from build123d import *

# Parameters (mm, degrees)
F1_DEPTH = 2
F2_DEPTH = 8
F3_DEPTH = 7.25


with BuildPart() as f1:
    # F0 (on Top) → F1 (new body)
    with BuildSketch(Plane.XY):
        with BuildLine():
            Line((4.85, 7.2), (-4.85, 7.2))
            ThreePointArc((-4.85, 7.2), (-6.5117009358, 6.5117009358), (-7.2, 4.85))
            Line((-7.2, 4.85), (-7.2, -4.85))
            ThreePointArc((-7.2, -4.85), (-6.5117009358, -6.5117009358), (-4.85, -7.2))
            Line((-4.85, -7.2), (4.85, -7.2))
            ThreePointArc((4.85, -7.2), (6.5117009358, -6.5117009358), (7.2, -4.85))
            Line((7.2, -4.85), (7.2, 4.85))
            ThreePointArc((7.2, 4.85), (6.5117009358, 6.5117009358), (4.85, 7.2))
        make_face()
        with BuildLine():
            ThreePointArc((6.45, -4.85), (5.9813708499, -5.9813708499), (4.85, -6.45))
            Line((4.85, -6.45), (-4.85, -6.45))
            ThreePointArc((-4.85, -6.45), (-5.9813708499, -5.9813708499), (-6.45, -4.85))
            Line((-6.45, -4.85), (-6.45, 4.85))
            ThreePointArc((-6.45, 4.85), (-5.9813708499, 5.9813708499), (-4.85, 6.45))
            Line((-4.85, 6.45), (4.85, 6.45))
            ThreePointArc((4.85, 6.45), (5.9813708499, 5.9813708499), (6.45, 4.85))
            Line((6.45, 4.85), (6.45, -4.85))
        make_face(mode=Mode.SUBTRACT)
    extrude(amount=F1_DEPTH)

    # F0 (on Top) → F2 (join)
    with BuildSketch(Plane.XY):
        with BuildLine():
            Line((-4.85, -6.45), (4.85, -6.45))
            ThreePointArc((4.85, -6.45), (5.9813708499, -5.9813708499), (6.45, -4.85))
            Line((6.45, -4.85), (6.45, 4.85))
            ThreePointArc((6.45, 4.85), (5.9813708499, 5.9813708499), (4.85, 6.45))
            Line((4.85, 6.45), (-4.85, 6.45))
            ThreePointArc((-4.85, 6.45), (-5.9813708499, 5.9813708499), (-6.45, 4.85))
            Line((-6.45, 4.85), (-6.45, -4.85))
            ThreePointArc((-6.45, -4.85), (-5.9813708499, -5.9813708499), (-4.85, -6.45))
        make_face()
        Polygon((1.355533, 3.320697), (-0.67179, 0.676571), (-0.439293, 0.773395), (-0.210383, 0.843921), (0.016137, 0.886954), (0.241462, 0.901298), (0.470596, 0.891361), (0.689421, 0.861552), (0.897936, 0.81187), (1.096141, 0.742316), (1.284036, 0.652888), (1.461621, 0.543588), (1.628896, 0.414415), (1.785861, 0.265369), (1.928183, 0.100858), (2.051528, -0.07471), (2.155898, -0.261335), (2.241291, -0.459016), (2.307708, -0.667755), (2.355149, -0.887551), (2.383613, -1.118404), (2.393101, -1.360314), (2.382455, -1.62389), (2.350517, -1.874317), (2.297286, -2.111595), (2.222763, -2.335724), (2.126948, -2.546704), (2.00984, -2.744536), (1.871441, -2.929218), (1.711749, -3.100751), (1.534649, -3.2554), (1.344027, -3.38943), (1.139883, -3.502839), (0.922217, -3.595628), (0.691027, -3.667798), (0.446316, -3.719348), (0.188082, -3.750277), (-0.083675, -3.760587), (-0.337875, -3.750502), (-0.579299, -3.720244), (-0.807948, -3.669815), (-1.023822, -3.599214), (-1.22692, -3.508442), (-1.417243, -3.397498), (-1.594791, -3.266383), (-1.759563, -3.115096), (-1.908048, -2.947372), (-2.036736, -2.766948), (-2.145625, -2.573824), (-2.234717, -2.367999), (-2.30401, -2.149473), (-2.353505, -1.918246), (-2.383202, -1.674319), (-2.393101, -1.417691), (-2.387124, -1.273221), (-2.369194, -1.12072), (-2.33931, -0.960188), (-2.297473, -0.791624), (-2.243682, -0.615029), (-2.177937, -0.430403), (-2.100239, -0.237745), (-2.010587, -0.037056), (-1.795423, 0.388416), (-1.532445, 0.846013), (-1.221653, 1.335735), (-0.863046, 1.857582), (-0.73873, 2.024932), (0.485314, 3.760587), align=None, mode=Mode.SUBTRACT)
    extrude(amount=F2_DEPTH)



with BuildPart() as f2:
    # F0 (on Top) → F2, piece 2 (new body)
    with BuildSketch(Plane.XY):
        Polygon((-1.302227, -1.275519), (-1.307719, -1.427254), (-1.302265, -1.580035), (-1.285903, -1.725196), (-1.258634, -1.862737), (-1.220458, -1.992657), (-1.171373, -2.114957), (-1.111381, -2.229636), (-1.040482, -2.336695), (-0.958675, -2.436134), (-0.868201, -2.525786), (-0.771303, -2.603484), (-0.667979, -2.669228), (-0.558231, -2.723019), (-0.442057, -2.764857), (-0.319459, -2.79474), (-0.190435, -2.812671), (-0.054986, -2.818648), (0.097421, -2.81282), (0.241462, -2.795338), (0.377135, -2.766201), (0.50444, -2.72541), (0.623378, -2.672964), (0.733948, -2.608863), (0.836151, -2.533107), (0.929986, -2.445697), (1.014035, -2.348201), (1.086877, -2.242188), (1.148512, -2.127658), (1.198941, -2.004611), (1.238164, -1.873047), (1.26618, -1.732966), (1.28299, -1.584369), (1.288593, -1.427254), (1.283064, -1.267936), (1.266479, -1.117508), (1.238836, -0.97597), (1.200137, -0.843323), (1.15038, -0.719566), (1.089566, -0.6047), (1.017696, -0.498725), (0.934768, -0.401639), (0.842053, -0.314789), (0.740821, -0.239519), (0.631073, -0.175829), (0.512807, -0.123719), (0.386025, -0.083189), (0.250726, -0.054239), (0.10691, -0.036869), (-0.045423, -0.031079), (-0.18203, -0.037131), (-0.312137, -0.055285), (-0.435744, -0.085543), (-0.552852, -0.127903), (-0.663459, -0.182366), (-0.767567, -0.248933), (-0.865176, -0.327602), (-0.956284, -0.418374), (-1.038652, -0.518859), (-1.110037, -0.626665), (-1.17044, -0.741793), (-1.21986, -0.864242), (-1.258298, -0.994013), (-1.285754, -1.131105), align=None)
    extrude(amount=F2_DEPTH)


with BuildPart() as f1_1:
    add(f1.part)

    add(f2.part)  # F3 merges F2
    # F0 (on Top) → F3 (join)
    with BuildSketch(Plane.XY):
        Polygon((-0.439293, 0.773395), (-0.67179, 0.676571), (1.355533, 3.320697), (0.485314, 3.760587), (-0.73873, 2.024932), (-0.863046, 1.857582), (-1.221653, 1.335735), (-1.532445, 0.846013), (-1.795423, 0.388416), (-2.010587, -0.037056), (-2.100239, -0.237745), (-2.177937, -0.430403), (-2.243682, -0.615029), (-2.297473, -0.791624), (-2.33931, -0.960188), (-2.369194, -1.12072), (-2.387124, -1.273221), (-2.393101, -1.417691), (-2.383202, -1.674319), (-2.353505, -1.918246), (-2.30401, -2.149473), (-2.234717, -2.367999), (-2.145625, -2.573824), (-2.036736, -2.766948), (-1.908048, -2.947372), (-1.759563, -3.115096), (-1.594791, -3.266383), (-1.417243, -3.397498), (-1.22692, -3.508442), (-1.023822, -3.599214), (-0.807948, -3.669815), (-0.579299, -3.720244), (-0.337875, -3.750502), (-0.083675, -3.760587), (0.188082, -3.750277), (0.446316, -3.719348), (0.691027, -3.667798), (0.922217, -3.595628), (1.139883, -3.502839), (1.344027, -3.38943), (1.534649, -3.2554), (1.711749, -3.100751), (1.871441, -2.929218), (2.00984, -2.744536), (2.126948, -2.546704), (2.222763, -2.335724), (2.297286, -2.111595), (2.350517, -1.874317), (2.382455, -1.62389), (2.393101, -1.360314), (2.383613, -1.118404), (2.355149, -0.887551), (2.307708, -0.667755), (2.241291, -0.459016), (2.155898, -0.261335), (2.051528, -0.07471), (1.928183, 0.100858), (1.785861, 0.265369), (1.628896, 0.414415), (1.461621, 0.543588), (1.284036, 0.652888), (1.096141, 0.742316), (0.897936, 0.81187), (0.689421, 0.861552), (0.470596, 0.891361), (0.241462, 0.901298), (0.016137, 0.886954), (-0.210383, 0.843921), align=None)
        Polygon((-1.302265, -1.580035), (-1.307719, -1.427254), (-1.302227, -1.275519), (-1.285754, -1.131105), (-1.258298, -0.994013), (-1.21986, -0.864242), (-1.17044, -0.741793), (-1.110037, -0.626665), (-1.038652, -0.518859), (-0.956284, -0.418374), (-0.865176, -0.327602), (-0.767567, -0.248933), (-0.663459, -0.182366), (-0.552852, -0.127903), (-0.435744, -0.085543), (-0.312137, -0.055285), (-0.18203, -0.037131), (-0.045423, -0.031079), (0.10691, -0.036869), (0.250726, -0.054239), (0.386025, -0.083189), (0.512807, -0.123719), (0.631073, -0.175829), (0.740821, -0.239519), (0.842053, -0.314789), (0.934768, -0.401639), (1.017696, -0.498725), (1.089566, -0.6047), (1.15038, -0.719566), (1.200137, -0.843323), (1.238836, -0.97597), (1.266479, -1.117508), (1.283064, -1.267936), (1.288593, -1.427254), (1.28299, -1.584369), (1.26618, -1.732966), (1.238164, -1.873047), (1.198941, -2.004611), (1.148512, -2.127658), (1.086877, -2.242188), (1.014035, -2.348201), (0.929986, -2.445697), (0.836151, -2.533107), (0.733948, -2.608863), (0.623378, -2.672964), (0.50444, -2.72541), (0.377135, -2.766201), (0.241462, -2.795338), (0.097421, -2.81282), (-0.054986, -2.818648), (-0.190435, -2.812671), (-0.319459, -2.79474), (-0.442057, -2.764857), (-0.558231, -2.723019), (-0.667979, -2.669228), (-0.771303, -2.603484), (-0.868201, -2.525786), (-0.958675, -2.436134), (-1.040482, -2.336695), (-1.111381, -2.229636), (-1.171373, -2.114957), (-1.220458, -1.992657), (-1.258634, -1.862737), (-1.285903, -1.725196), align=None, mode=Mode.SUBTRACT)
    extrude(amount=F3_DEPTH)


solid = f1_1.part
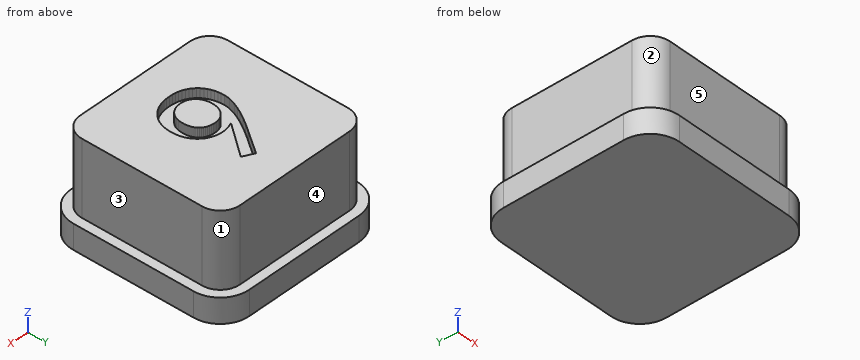
Geometry check sheet. Reference: the model listing, model coordinates, mm. Face numbers are marked on the shaded views. A direction names the side the tool comes from. Coordinates: 2 decimals unless noted, no trailing zeros. Order: outer loops, then holes, each group sorted by start corner. A loop starts at its lowest first (then second) coordinate and runs counter-clockwise, first axis right, second up. Notation, with made-up numbers: (29, 6.5) -> (54, 6.5) arc R24 cw to (54, 40.5) -> close; hole circle Ø9 at (36, 4.5). An arc over 180 degrees is marked (long way). Use a Markdown table: item, result. Add a question column.
1. Cross-section at A-A (z = 5.25). Enter the section's corners in (x, y).
2. Cross-section at C-C (y = 2.25). Enter the section's corners in (x, z), and give its area (3 significant figures).
3. Cross-section at B-B (x = 2.75). Enter the section's corners in (y, z), and give its area (3 significant figures).
4. Set-up check for the marked faces 1, 2, 3, 4 and 5: record each of +Z, -Z, +X, -X, +Y, -Y from which the full face is reachable in a straight line by a thin tool's end or side.
5. Material ranges on L1, parallel to X at y = 0.5, z = 6; L2, parallel to Z at x = 6.75, y = 2.25, recorded low to high.
6. Go/stop test with flat-tipped pins: pin 1 Ø1 at (x, z) = (-2.5, 7) entering from +Y; pin 2 Ø6 at (x, y) = (-3.5, 4) entering from -Z; pin 3 Ø1.8 at (y, z) = (0, 4.5) entering from -X; pin 4 Ø1.5 at (y, z) = (3, 4) entering from +X. Record where each tip stops, or that it passes through.
Filled sheet:
| question | item | result |
|---|---|---|
| 1 | outline | (-6.45, -4.85) arc R1.6 ccw to (-4.85, -6.45) -> (4.85, -6.45) arc R1.6 ccw to (6.45, -4.85) -> (6.45, 4.85) arc R1.6 ccw to (4.85, 6.45) -> (-4.85, 6.45) arc R1.6 ccw to (-6.45, 4.85) -> close |
| 2 | outline | (-7.2, 0) -> (7.2, 0) -> (7.2, 2) -> (6.45, 2) -> (6.45, 8) -> (0.53, 8) -> (0.53, 7.25) -> (-0.58, 7.25) -> (-0.58, 8) -> (-6.45, 8) -> (-6.45, 2) -> (-7.2, 2) -> close |
| 2 | area | 105 mm2 |
| 3 | outline | (-7.2, 0) -> (7.2, 0) -> (7.2, 2) -> (6.45, 2) -> (6.45, 8) -> (-6.45, 8) -> (-6.45, 2) -> (-7.2, 2) -> close |
| 3 | area | 106 mm2 |
| 4 | face 1 | +Z, +X, +Y |
| 4 | face 2 | +Z, -X, -Y |
| 4 | face 3 | +Z, +X, +Y, -Y |
| 4 | face 4 | +Z, +X, -X, +Y |
| 4 | face 5 | +Z, +X, -X, -Y |
| 5 | L1 | -6.45 to 6.45 |
| 5 | L2 | 0 to 2 |
| 6 | pin 1 | y = 6.45 |
| 6 | pin 2 | z = 0 |
| 6 | pin 3 | x = -6.45 |
| 6 | pin 4 | x = 6.45 |
